```python
from build123d import *

# Parameters (mm, degrees)
BOSS_EXTRUDE1_DEPTH = 1.8
SKETCH4_W           = 44.55
SKETCH4_H           = 1.8
BOSS_EXTRUDE2_DEPTH = 4


with BuildPart() as part:
    # Sketch2 → Boss-Extrude1 (new body)
    with BuildSketch(Plane(origin=(0, 0, 0), x_dir=(1, 0, 0), z_dir=(0, 1, 0))):
        with BuildLine():
            Line((-32.275, 7.2), (32.275, 7.2))
            Line((32.275, 7.2), (32.275, 5.8))
            ThreePointArc((32.275, 5.8), (29.476225417, -2.258225611), (22.285, -6.846734756))
            Line((22.285, -6.846734756), (22.285, -2.012121212))
            ThreePointArc((22.285, -2.012121212), (21.992106781, -1.305014431), (21.285, -1.012121212))
            Line((21.285, -1.012121212), (20.485, -1.012121212))
            ThreePointArc((20.485, -1.012121212), (19.777893219, -1.305014431), (19.485, -2.012121212))
            Line((19.485, -2.012121212), (19.485, -7.198303735))
            ThreePointArc((19.485, -7.198303735), (19.380003425, -7.199575927), (19.275, -7.2))
            Line((19.275, -7.2), (15.325, -7.2))
            Line((15.325, -7.2), (15.325, -1.543434343))
            ThreePointArc((15.325, -1.543434343), (15.032106781, -0.836327562), (14.325, -0.543434343))
            Line((14.325, -0.543434343), (13.525, -0.543434343))
            ThreePointArc((13.525, -0.543434343), (12.817893219, -0.836327562), (12.525, -1.543434343))
            Line((12.525, -1.543434343), (12.525, -7.2))
            Line((12.525, -7.2), (8.365, -7.2))
            Line((8.365, -7.2), (8.365, -1.074747475))
            ThreePointArc((8.365, -1.074747475), (8.072106781, -0.367640694), (7.365, -0.074747475))
            Line((7.365, -0.074747475), (6.565, -0.074747475))
            ThreePointArc((6.565, -0.074747475), (5.857893219, -0.367640694), (5.565, -1.074747475))
            Line((5.565, -1.074747475), (5.565, -7.2))
            Line((5.565, -7.2), (1.405, -7.2))
            Line((1.405, -7.2), (1.405, -0.606060606))
            ThreePointArc((1.405, -0.606060606), (1.112106781, 0.101046175), (0.405, 0.393939394))
            Line((0.405, 0.393939394), (-0.395, 0.393939394))
            ThreePointArc((-0.395, 0.393939394), (-1.102106781, 0.101046175), (-1.395, -0.606060606))
            Line((-1.395, -0.606060606), (-1.395, -7.2))
            Line((-1.395, -7.2), (-5.555, -7.2))
            Line((-5.555, -7.2), (-5.555, -0.137373737))
            ThreePointArc((-5.555, -0.137373737), (-5.847893219, 0.569733044), (-6.555, 0.862626263))
            Line((-6.555, 0.862626263), (-7.355, 0.862626263))
            ThreePointArc((-7.355, 0.862626263), (-8.062106781, 0.569733044), (-8.355, -0.137373737))
            Line((-8.355, -0.137373737), (-8.355, -7.2))
            Line((-8.355, -7.2), (-12.515, -7.2))
            Line((-12.515, -7.2), (-12.515, 0.331313131))
            ThreePointArc((-12.515, 0.331313131), (-12.807893219, 1.038419912), (-13.515, 1.331313131))
            Line((-13.515, 1.331313131), (-14.315, 1.331313131))
            ThreePointArc((-14.315, 1.331313131), (-15.022106781, 1.038419912), (-15.315, 0.331313131))
            Line((-15.315, 0.331313131), (-15.315, -7.2))
            Line((-15.315, -7.2), (-19.275, -7.2))
            ThreePointArc((-19.275, -7.2), (-19.375002959, -7.199615356), (-19.475, -7.198461447))
            Line((-19.475, -7.198461447), (-19.475, 0.8))
            ThreePointArc((-19.475, 0.8), (-19.767893219, 1.507106781), (-20.475, 1.8))
            Line((-20.475, 1.8), (-21.275, 1.8))
            ThreePointArc((-21.275, 1.8), (-21.982106781, 1.507106781), (-22.275, 0.8))
            Line((-22.275, 0.8), (-22.275, -6.849110641))
            ThreePointArc((-22.275, -6.849110641), (-29.473039027, -2.262257748), (-32.275, 5.8))
            Line((-32.275, 5.8), (-32.275, 7.2))
        make_face()
    extrude(amount=BOSS_EXTRUDE1_DEPTH)

    # Sketch4 → Boss-Extrude2 (add)
    with BuildSketch(Plane(origin=(0, 1.8, 0), x_dir=(1, 0, 0), z_dir=(0, 1, 0))):
        with Locations((0, 6.3)):
            Rectangle(SKETCH4_W, SKETCH4_H)
    extrude(amount=BOSS_EXTRUDE2_DEPTH)


solid = part.part
```
Here's how the part is built. I have some questions about the finished solid (model axes, mm). A direction names the side the tool comes from. Give positions to 0.01 mm unless a question says otherwise; leave off trailing zeros. Order: outer loops, then holes, each group sorted by start corner. A loop starts at its lowest first (then second) coordinate and runs counter-clockwise, first axis right, second up. Notation, with made-up numbers: M 70.5,49 L 102.5,49 A20 cw 102.5,57 Z; hole C 78,45 d8. An arc over 180 degrees is marked long. Use a Markdown table: item, result. Add a question column.
1. If we mould it in two halves opening along X, with no side actions, what happens to faces 4 (the flat face through (0, 1.8, -3)), 5 (the cylindrical face through (-29.397, 0.887, 2.357)), 6 (the flat face through (19.485, 1, 5))? For each: +X half, -X half, draft (parallel to the pull), parting line (faces both ways), or undercut.
2. For pin 1 Ø0.5 at (y, z) = (1, 3.5) entering from -X; pin 2 Ø0.9 at (y, z) = (1, 3) entering from -X; pin 3 Ø0.9 at (x, y) = (20.5, 1) entering from +Z, each with a flat end and sliding along its axis, tell me the tip position at first contact or that it passes through.
3. I need wall thicknesses on probe 1 along X at (y, z) = (0.2, 0.5) (3 decimals); probe 2 along Y at (x, z) = (-28.5, 0.25); probe 3 along Z at (x, y) = (-15, 3.1). Which ranges of each line are inside material? Lowest first, please. Write a range as from..to.
4. Suppose I cut it at A-A (z = 2.75). Give the number of separate pieces and of enclosed holes in the cut face, and give its area (3 significant figures).
5. Suppose I cut it at D-D (x = -24.5). List the corners of the cut face in (y, z) for me.
6. Suppose I cut it at B-B (y = 2.8). List the corners of the cut face in (x, z) for me (3 decimals), and give its area (3 significant figures).
7. On a 3-axis mill with a long thin cutter (end or side, diameter ignored), from which of +Z, -Z, +X, -X, +Y, -Y can I reach the whole of each face in a straight line? I mean faces 1 (the cylindrical face through (19.786, 0.887, 1.297)), 2 (the flat face through (4, 1, 7.2)), 3 (the flat face through (0, 4, -5.4)). Say none if no direction works.
Results list:
| question | item | result |
|---|---|---|
| 1 | face 4 | draft |
| 1 | face 5 | -X half |
| 1 | face 6 | undercut |
| 2 | pin 1 | stops at x = -28.61 |
| 2 | pin 2 | stops at x = -29.24 |
| 2 | pin 3 | stops at z = 1.11 |
| 3 | probe 1 | x = -30.646..-22.275, -19.475..-15.315, -12.515..-8.355, -5.555..-1.389, 1.399..5.747, 8.183..30.646 |
| 3 | probe 2 | y = 0..1.8 |
| 3 | probe 3 | z = -7.2..-5.4 |
| 4 | separate pieces | 8 |
| 4 | enclosed holes | 0 |
| 4 | area | 69.4 mm² |
| 5 | outline | M 0,-7.2 L 1.8,-7.2 L 1.8,6.1 L 0,6.1 Z |
| 6 | outline | M -22.275,-7.2 L 22.275,-7.2 L 22.275,-5.4 L -22.275,-5.4 Z |
| 6 | area | 80.2 mm² |
| 7 | face 1 | +Z, +Y, -Y |
| 7 | face 2 | +Z, +X, -X, +Y, -Y |
| 7 | face 3 | +Z, +X, -X, +Y |
